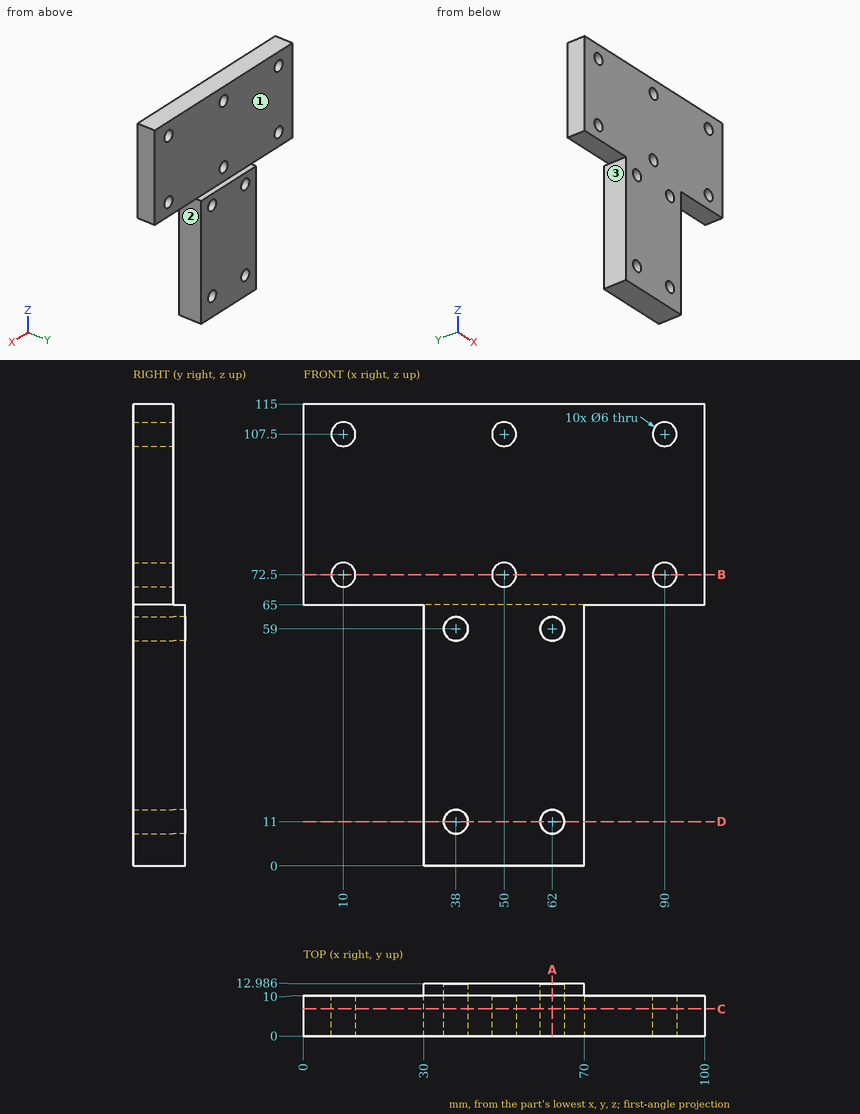
Answer from the drawing. Dimensions are ordinates in mm from the lowest x, y and z of the part. A direction names the side the tool comes from. Coordinates: 2 decimals unless noted, no trailing zeros. Write each loop counter-clockwise with the first axis right and the second up, starting at its lowest first coordinate (ties: lowest second). Pieces come first, ordered by that corner, then holes. Notation, with made-up numbers: M 47.25,72 L 67.25,72 A29 cw 67.25,97 Z; hole C 59.25,-25 d6. An arc over 180 degrees is marked long. Put each result on its own line as item: value. Start each with the question number.
1. A cutting plane is placed at B-B on z = 72.5. Write down the section's boundary in (x, y).
2. A cutting plane is placed at A-A on x = 62. Write down the section's boundary in (y, z).
3. Which of the six approach directions +Z, -Z, +X, -X, +Y, -Y give full straight-line access (tool end or side, diameter ignored) to the marked faces 1, 2 and 3?
4. A cutting plane is placed at C-C on y = 6.75. Count the separate pieces of the cut face and the enclosed holes in it, then the cut area to 3 significant figures.
5. Consider line 1 (Z direction, x = 50, y = 5.5); line 2 (Z direction, x = 90, y = 3.75); line 3 (X direction, y = 2, z = 11). Determine where each line is inside the solid, lowest interval first. Write a range as from..to.
6. Flat-ended cylindrical pins translate along their axes: P1, Ø8, axis at x = 50, z = 72.5, coming from the +Y side; P2, Ø5, axis at x = 84, y = 4.5, coming from the -Z side; P3, Ø2, axis at y = 6, z = 17.5, coming from the +X side. Find the tip coordinate at first contact, or state that the pin passes through.
7. A cutting plane is placed at D-D on z = 11. Write down the section's boundary in (x, y), then the cut area to 3 significant figures.
Resolved:
1. outline: M 0,0 L 7,0 L 7,10 L 0,10 Z; M 13,0 L 47,0 L 47,10 L 13,10 Z; M 53,0 L 87,0 L 87,10 L 53,10 Z; M 93,0 L 100,0 L 100,10 L 93,10 Z
2. outline: M 0,0 L 12.99,0 L 12.99,8 L 0,8 Z; M 0,14 L 12.99,14 L 12.99,56 L 0,56 Z; M 0,62 L 12.99,62 L 12.99,65 L 10,65 L 10,115 L 0,115 Z
3. face 1: +Z, +X, -X, +Y
3. face 2: -Z, +X, +Y, -Y
3. face 3: -Z, -X, +Y, -Y
4. separate pieces: 1
4. enclosed holes: 10
4. area: 7,320 mm2
5. line 1: z = 0..69.5, 75.5..104.5, 110.5..115
5. line 2: z = 65..69.5, 75.5..104.5, 110.5..115
5. line 3: x = 30..35, 41..59, 65..70
6. P1: stops at y = 10
6. P2: stops at z = 65
6. P3: stops at x = 70
7. outline: M 30,0 L 35,0 L 35,12.99 L 30,12.99 Z; M 41,0 L 59,0 L 59,12.99 L 41,12.99 Z; M 65,0 L 70,0 L 70,12.99 L 65,12.99 Z
7. area: 364 mm2
